For this review, take the finished solid that the model builds, in its own axes (mm). A direction names the side the tool comes from. Round coordinates to 2 decimals unless told otherwise and drop trailing zeros. Write each loop counter-clockwise with the first axis right and the second up, starting at its lowest first coordinate (ties: lowest second). Pieces come first, ordered by that corner, then holes. Notation, with made-up numbers: (6, 52.5) -> (33, 52.5) arc R17 ccw to (33, 79.5) -> close; hole circle Ø5 at (10, -29). An arc over 180 degrees is marked (long way). Answer in a Markdown table with one row per item. Add a question column.
```python
from build123d import *

# Parameters (mm, degrees)
BOSS_EXTRUDE1_DEPTH = 20
CUT_EXTRUDE1_DEPTH  = 5


with BuildPart() as part:
    # Sketch1 → Boss-Extrude1 (new body)
    with BuildSketch(Plane(origin=(0, 0, 0), x_dir=(1, 0, 0), z_dir=(0, 1, 0))):
        with BuildLine():
            Line((-25, -37.5), (25, -37.5))
            ThreePointArc((25, -37.5), (32.071067812, -34.571067812), (35, -27.5))
            Line((35, -27.5), (35, 27.5))
            ThreePointArc((35, 27.5), (32.071067812, 34.571067812), (25, 37.5))
            Line((25, 37.5), (-25, 37.5))
            ThreePointArc((-25, 37.5), (-32.071067812, 34.571067812), (-35, 27.5))
            Line((-35, 27.5), (-35, -27.5))
            ThreePointArc((-35, -27.5), (-32.071067812, -34.571067812), (-25, -37.5))
        make_face()
        with BuildLine():
            Line((-21, -17.5), (-21, 17.5))
            ThreePointArc((-21, 17.5), (-16, 22.5), (-11, 17.5))
            Line((-11, 17.5), (-11, -17.5))
            ThreePointArc((-11, -17.5), (-16, -22.5), (-21, -17.5))
        make_face(mode=Mode.SUBTRACT)
        with BuildLine():
            Line((21, -17.5), (21, 17.5))
            ThreePointArc((21, 17.5), (16, 22.5), (11, 17.5))
            Line((11, 17.5), (11, -17.5))
            ThreePointArc((11, -17.5), (16, -22.5), (21, -17.5))
        make_face(mode=Mode.SUBTRACT)
    extrude(amount=BOSS_EXTRUDE1_DEPTH)

    # Sketch2 → Cut-Extrude1 (cut)
    with BuildSketch(Plane(origin=(0, 20, 0), x_dir=(1, 0, 0), z_dir=(0, 1, 0))):
        with BuildLine():
            Line((-16, -22.5), (16, -22.5))
            ThreePointArc((16, -22.5), (12.464466094, -21.035533906), (11, -17.5))
            Line((11, -17.5), (11, 17.5))
            ThreePointArc((11, 17.5), (12.464466094, 21.035533906), (16, 22.5))
            Line((16, 22.5), (-16, 22.5))
            ThreePointArc((-16, 22.5), (-12.464466094, 21.035533906), (-11, 17.5))
            Line((-11, 17.5), (-11, -17.5))
            ThreePointArc((-11, -17.5), (-12.464466094, -21.035533906), (-16, -22.5))
        make_face()
    extrude(amount=-CUT_EXTRUDE1_DEPTH, mode=Mode.SUBTRACT)


solid = part.part
```
1. Clearance check with a flat-ended pin moving along its axis: pin 1 Ø9.5 at (x, z) = (-1.5, -3.5) entering from +Y. State where the tip first meets the part, or that it passes through.
2. Tool access review of faces 1 (the flat face through (0, 18, -22.5)), 2 (the flat face through (-35, 10, 0)), 3 (the flat face through (11, 7, 0)): name each direction out of +Z, -Z, +X, -X, +Y, -Y from which nothing blocks a thin tool from reaching the whole face with its end or side.
3. We need section D-D (x = 7). Write out the cut boundary in (y, z), plus the area to 4 significant figures.
4. We need section A-A (z = -2.5). Write out the cut boundary in (x, y), plus the area to 3 significant figures.
5. The part is to be moulded in two halves that separate along X. For faces 4 (the cylindrical face through (-31.99, 9.86, -34.65)), 5 (the flat face through (23, 20, -1)), 6 (the cylindrical face through (16.1, 9.9, -22.5)), 7 (the flat face through (0, 15, 0)), say which applies: pulls with the +X half, pulls with the -X half, needs draft (parallel to the pull), parting line crosses it, or undercut.
6. For L1, parallel to X at y = 12.75, z = -12.5; L2, parallel to X at y = 2, z = -18.5; L3, parallel to Z at x = 3, y = 17.5, list the stretches that pass through material, from the lowest coordinate up. Write a range as [from, to].
7. We need section B-B (y = 17.25). Write out the cut boundary in (x, z).
8. We need section C-C (y = 4.75). Write out the cut boundary in (x, z), plus the area to 3 significant figures.
Response:
| question | item | result |
|---|---|---|
| 1 | pin 1 | y = 15 |
| 2 | face 1 | +Y |
| 2 | face 2 | +Z, -Z, -X, +Y, -Y |
| 2 | face 3 | +Y, -Y |
| 3 | outline | (0, -37.5) -> (20, -37.5) -> (20, -22.5) -> (15, -22.5) -> (15, 22.5) -> (20, 22.5) -> (20, 37.5) -> (0, 37.5) -> close |
| 3 | area | 1,275 mm2 |
| 4 | outline | (-35, 0) -> (-21, 0) -> (-21, 20) -> (-35, 20) -> close; (-11, 0) -> (11, 0) -> (11, 15) -> (-11, 15) -> close; (21, 0) -> (35, 0) -> (35, 20) -> (21, 20) -> close |
| 4 | area | 890 mm2 |
| 5 | face 4 | pulls with the -X half |
| 5 | face 5 | needs draft |
| 5 | face 6 | undercut |
| 5 | face 7 | undercut |
| 6 | L1 | [-35, -21], [-11, 11], [21, 35] |
| 6 | L2 | [-35, -20.9], [-11.1, 11.1], [20.9, 35] |
| 6 | L3 | [-37.5, -22.5], [22.5, 37.5] |
| 7 | outline | (-35, -27.5) arc R10 ccw to (-25, -37.5) -> (25, -37.5) arc R10 ccw to (35, -27.5) -> (35, 27.5) arc R10 ccw to (25, 37.5) -> (-25, 37.5) arc R10 ccw to (-35, 27.5) -> close; hole (-21, -17.5) arc R5 ccw to (-16, -22.5) -> (16, -22.5) arc R5 ccw to (21, -17.5) -> (21, 17.5) arc R5 ccw to (16, 22.5) -> (-16, 22.5) arc R5 ccw to (-21, 17.5) -> close |
| 8 | outline | (-35, -27.5) arc R10 ccw to (-25, -37.5) -> (25, -37.5) arc R10 ccw to (35, -27.5) -> (35, 27.5) arc R10 ccw to (25, 37.5) -> (-25, 37.5) arc R10 ccw to (-35, 27.5) -> close; hole (-21, -17.5) arc R5 ccw to (-11, -17.5) -> (-11, 17.5) arc R5 ccw to (-21, 17.5) -> close; hole (11, -17.5) arc R5 ccw to (21, -17.5) -> (21, 17.5) arc R5 ccw to (11, 17.5) -> close |
| 8 | area | 4,310 mm2 |
